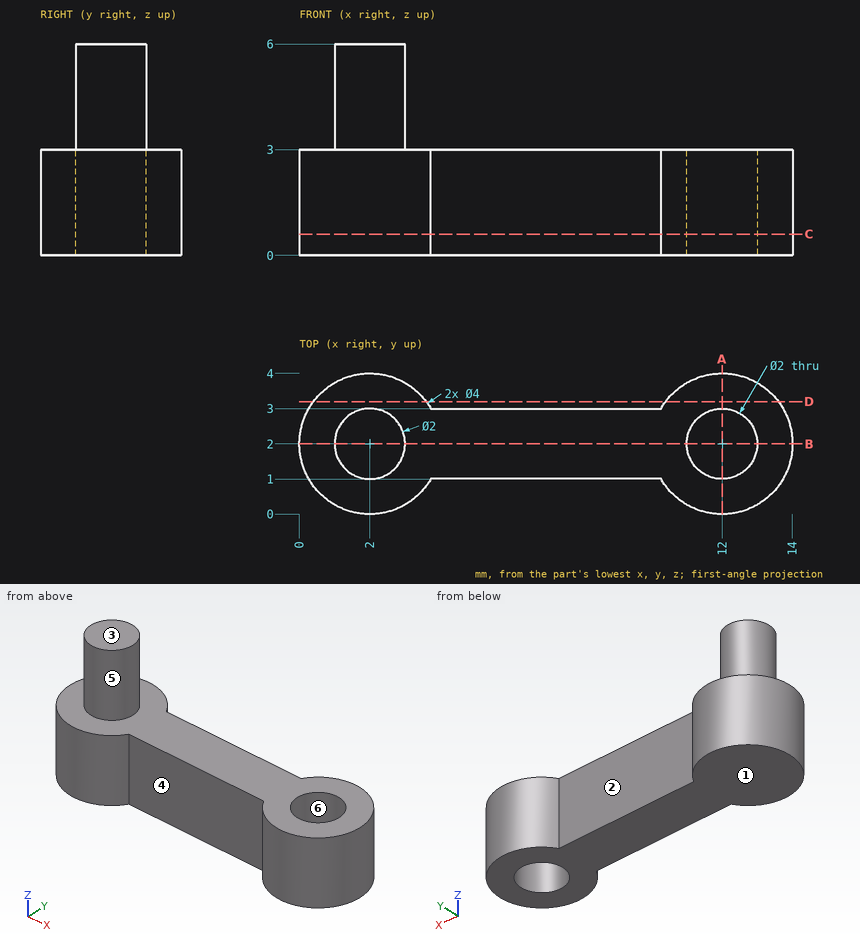
Print and shaded views of the part. All mm, measured from the part's lowest x, y and z. A direction names the side the tool comes from. Round coordinates to 2 decimals unless told otherwise and drop trailing zeros. Write each loop counter-clockwise with the first axis right and the second up, starting at its lowest first coordinate (ties: lowest second). Pieces come first, ordered by that corner, then holes.
(1) Slice it at B-B, the plane y = 2. Write the cut outline in (x, z), and give its area (3 significant figures).
(2) Slice it at D-D, the plane y = 3.2. Write the cut outline in (x, z), and give its area (3 significant figures).
(3) Slice it at C-C, the plane z = 0.6. Write the cut outline in (x, y).
(4) Drop flat-ended pins along their axis: P1, Ø1, axis at x = 4, z = 2, coming from the +Y side; P2, Ø2, axis at x = 8.5, y = 3, coming from the +Z side; P3, Ø2.5, axis at x = 7, z = 1.5, coming from the +Y side. Give the stop position or say it passes through.
(5) 3-axis set-ups, long thin cutter, end or side, ignore diameter. For the marked faces 1 and 2: which of +Z, -Z, +X, -X, +Y, -Y reach the whole face in a straight line?
(6) Mould opens along Y. For the marked faces 3, 4, 5 and 6 say: pulls with the +Y half, pulls with the -Y half, needs draft (parallel to the pull), parting line crosses it, or undercut.
(7) Probe line 1 along Y through (x, z) = (12, 1); line 2 along Z through (x, y) = (13.5, 1.5); line 3 along Y through (x, z) = (5.25, 0.8). List the from-to ranges inside material, lowest first.
(8) Slice it at A-A, the plane x = 12. Write the cut outline in (y, z), and give its area (3 significant figures).
From the geometry:
1. outline: (0, 0) - (11, 0) - (11, 3) - (3, 3) - (3, 6) - (1, 6) - (1, 3) - (0, 3) - close; (13, 0) - (14, 0) - (14, 3) - (13, 3) - close
1. area: 42.0 mm2
2. outline: (0.4, 0) - (3.6, 0) - (3.6, 3) - (0.4, 3) - close; (10.4, 0) - (13.6, 0) - (13.6, 3) - (10.4, 3) - close
2. area: 19.2 mm2
3. outline: (3.73, 1) - (10.27, 1) arc R2 ccw (long way) to (10.27, 3) - (3.73, 3) arc R2 ccw (long way) to start; hole circle Ø2 at (12, 2)
4. P1: stops at y = 3.32
4. P2: stops at z = 3
4. P3: stops at y = 3
5. face 1: -Z, +X, -X, +Y, -Y
5. face 2: +Z, -Z, +Y
6. face 3: needs draft
6. face 4: pulls with the -Y half
6. face 5: parting line crosses it
6. face 6: undercut
7. line 1: y = 0 to 1, 3 to 4
7. line 2: z = 0 to 3
7. line 3: y = 1 to 3
8. outline: (0, 0) - (1, 0) - (1, 3) - (0, 3) - close; (3, 0) - (4, 0) - (4, 3) - (3, 3) - close
8. area: 6.00 mm2
